Study the drawing (mm; zero at the part's minimum x, y, z) and answer. A direction names the side the tool comes from. Give positions to 0.01 mm unless a question says otherwise; leave off trailing zeros. Order: outer loops, then holes, each group sorted by start corner. A loop starts at its lowest first (then second) coordinate and runs counter-clockwise, first axis right, second up.
Item 1: The mould has two halves that part along Y. Classify the marked faces 1, 2, 3 and 4: +Y half, -Y half, draft (parallel to the pull), parting line (faces both ways), or undercut.
Item 2: A cutting plane is placed at D-D (y = 27.94). Write down the section's boundary in (x, z) (1 decimal), plus the area to 3 significant figures.
Item 3: Which of the six approach directions +Z, -Z, +X, -X, +Y, -Y give full straight-line access (tool end or side, diameter ignored) to the marked faces 5, 6 and 7?
Item 4: A cutting plane is placed at C-C (y = 4). Write down the section's boundary in (x, z), plus the area to 3 significant figures.
Item 5: A cutting plane is placed at A-A (z = 11.75). Write down the section's boundary in (x, y).
Item 6: Find the intervals of material crossed by line 1 along Y through (x, z) = (7, 14.25); line 2 along Y through (x, z) = (2.5, 14); line 3 along Y through (x, z) = (11.25, 18.25), in increasing order.
Item 7: A cutting plane is placed at B-B (x = 2.75). State how many separate pieces and enclosed holes the cut face has.
Item 8: Given pin 1 Ø3.5 at (y, z) = (52, 16) entering from +X; pin 2 Ø1.5 at (x, y) = (13.5, 23.5) entering from -Z; pin 3 Ø4.5 at (x, y) = (11.5, 15) entering from +Z; pin 4 Ø3 at (x, y) = (8, 27.5) entering from -Z, each flat-ended and moving along its own axis, determine where each tip first touches the part or whether it passes through.
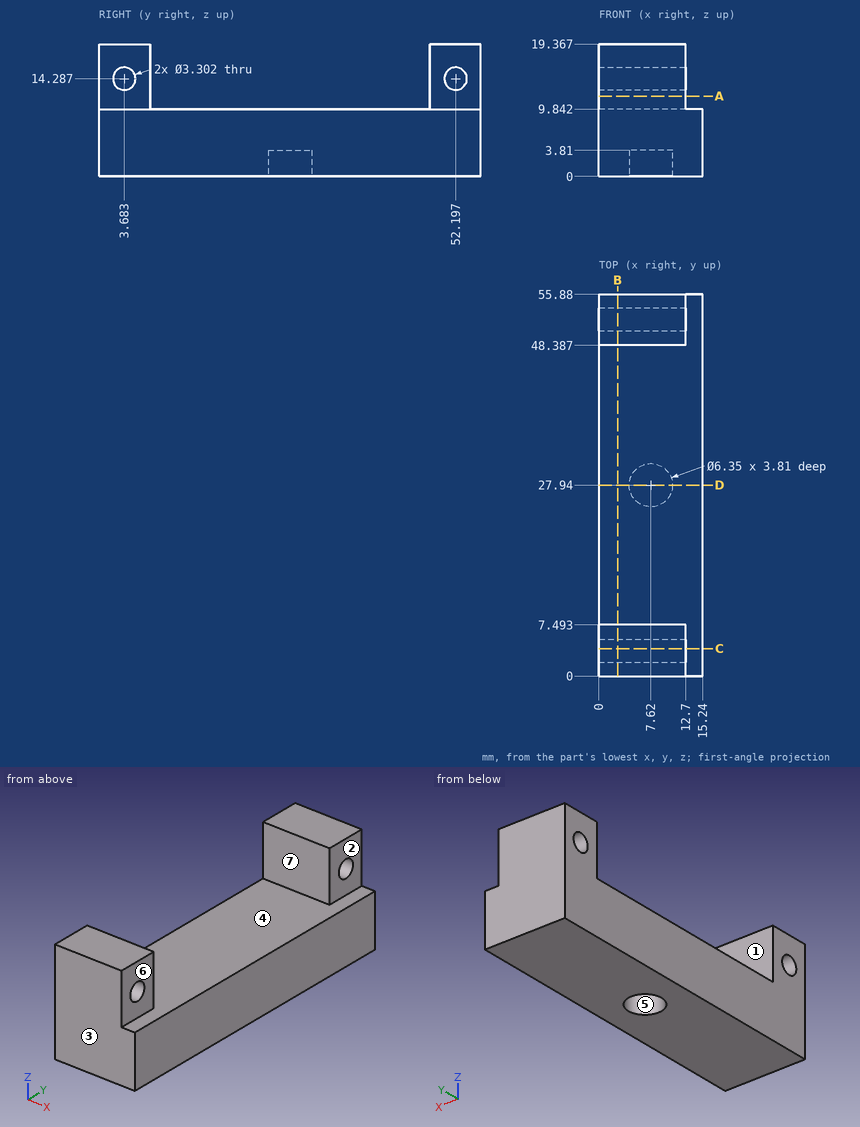
Response values:
1. face 1: undercut
1. face 2: draft
1. face 3: -Y half
1. face 4: undercut
2. outline: (0, 0) - (4.4, 0) - (4.4, 3.8) - (10.8, 3.8) - (10.8, 0) - (15.2, 0) - (15.2, 9.8) - (0, 9.8) - close
2. area: 126 mm2
3. face 5: -Z
3. face 6: +Z, +X, +Y, -Y
3. face 7: +Z, +X, -X
4. outline: (0, 0) - (15.24, 0) - (15.24, 9.84) - (12.7, 9.84) - (12.7, 12.67) - (0, 12.67) - close; (0, 15.91) - (12.7, 15.91) - (12.7, 19.37) - (0, 19.37) - close
4. area: 230 mm2
5. outline: (0, 0) - (12.7, 0) - (12.7, 7.49) - (0, 7.49) - close; (0, 48.39) - (12.7, 48.39) - (12.7, 55.88) - (0, 55.88) - close
6. line 1: y = 0 to 2.03, 5.33 to 7.49, 48.39 to 50.55, 53.85 to 55.88
6. line 2: y = 0 to 2.06, 5.31 to 7.49, 48.39 to 50.57, 53.82 to 55.88
6. line 3: y = 0 to 7.49, 48.39 to 55.88
7. separate pieces: 1
7. enclosed holes: 2
8. pin 1: stops at x = 12.7
8. pin 2: stops at z = 0
8. pin 3: stops at z = 9.84
8. pin 4: stops at z = 3.81
